Geometry check sheet. Reference: the model listing, model coordinates, mm. Face numbers are marked on the shaded views. A direction names the side the tool comes from. Round coordinates to 2 decimals unless told otherwise and drop trailing zeros. Loops run counter-clockwise (first coordinate to the right, second up) from the corner with the lowest first, then second, coordinate; pieces in that order, holes last.
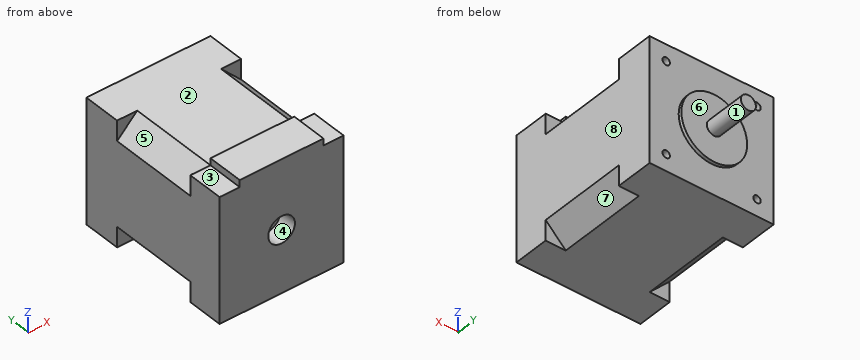
```python
from build123d import *

# Parameters (mm, degrees)
SKETCH1_W               = 41.45
SKETCH1_H               = 41.45
BOSS_EXTRUDE1_DEPTH     = 54.6
SKETCH2_R               = 11
BOSS_EXTRUDE2_DEPTH     = 1.1
SKETCH3_R               = 2.5
BOSS_EXTRUDE3_DEPTH     = 14
BOSS_EXTRUDE4_DEPTH     = 12
SKETCH5_R               = 1.25
CUT_EXTRUDE1_DEPTH      = 12
MIRROR2_COPY_1_SKETCH_R = 1.25
MIRROR2_COPY_1_DEPTH    = 12
CUT_EXTRUDE2_DEPTH      = 30
MIRROR4_COPY_1_DEPTH    = 30
SKETCH10_R              = 4.45
CUT_EXTRUDE3_DEPTH      = 6


with BuildPart() as part:
    # Sketch1 → Boss-Extrude1 (new body)
    with BuildSketch(Plane(origin=(0, 0, 0), x_dir=(1, 0, 0), z_dir=(0, 1, 0))):
        Rectangle(SKETCH1_W, SKETCH1_H)
    extrude(amount=BOSS_EXTRUDE1_DEPTH)

    # Sketch2 → Boss-Extrude2 (add)
    with BuildSketch(Plane(origin=(0, 54.6, 0), x_dir=(1, 0, 0), z_dir=(0, 1, 0))):
        Circle(SKETCH2_R)
    extrude(amount=BOSS_EXTRUDE2_DEPTH)

    # Sketch3 → Boss-Extrude3 (add)
    with BuildSketch(Plane(origin=(0, 55.7, 0), x_dir=(1, 0, 0), z_dir=(0, 1, 0))):
        Circle(SKETCH3_R)
    extrude(amount=BOSS_EXTRUDE3_DEPTH)

    # Sketch4 → Boss-Extrude4 (add)
    with BuildSketch(Plane.XZ):
        Polygon((0, 20.725), (14, 20.725), (14, 23.025), (-14, 23.025), (-14, 20.725), align=None)
    extrude(amount=-BOSS_EXTRUDE4_DEPTH)

    # Sketch5 → Cut-Extrude1 (cut)
    with BuildSketch(Plane(origin=(0, 54.6, 0), x_dir=(1, 0, 0), z_dir=(0, 1, 0))):
        with Locations((15.175, 15.175)):
            Circle(SKETCH5_R)
    cut_extrude1 = extrude(amount=-CUT_EXTRUDE1_DEPTH, mode=Mode.SUBTRACT)

    # Mirror1: Cut-Extrude1 across plane
    add(cut_extrude1.mirror(Plane.XY), mode=Mode.SUBTRACT)

    # Mirror2: Cut-Extrude1 across plane
    add(cut_extrude1.mirror(Plane(origin=(0, 0, 0), x_dir=(0, 0, 1), z_dir=(1, 0, 0))), mode=Mode.SUBTRACT)

    # Mirror2 copy 1 sketch → Mirror2 copy 1 (cut)
    with BuildSketch(Plane(origin=(0, 54.6, 0), x_dir=(-1, 0, 0), z_dir=(0, 1, 0))):
        with Locations((15.175, 15.175)):
            Circle(MIRROR2_COPY_1_SKETCH_R)
    extrude(amount=-MIRROR2_COPY_1_DEPTH, mode=Mode.SUBTRACT)

    # Sketch8 → Cut-Extrude2 (cut)
    with BuildSketch(Plane(origin=(0, 12, 0), x_dir=(1, 0, 0), z_dir=(0, 1, 0))):
        Polygon((-20.725, 14), (-20.725, 20.725), (-14, 20.725), align=None)
    cut_extrude2 = extrude(amount=CUT_EXTRUDE2_DEPTH, mode=Mode.SUBTRACT)

    # Mirror3: Cut-Extrude2 across plane
    add(cut_extrude2.mirror(Plane(origin=(0, 0, 0), x_dir=(0, 0, 1), z_dir=(1, 0, 0))), mode=Mode.SUBTRACT)

    # Mirror4: Cut-Extrude2 across plane
    add(cut_extrude2.mirror(Plane.XY), mode=Mode.SUBTRACT)

    # Mirror4 copy 1 sketch → Mirror4 copy 1 (cut)
    with BuildSketch(Plane(origin=(0, 12, 0), x_dir=(-1, 0, 0), z_dir=(0, 1, 0))):
        Polygon((-20.725, 14), (-20.725, 20.725), (-14, 20.725), align=None)
    extrude(amount=MIRROR4_COPY_1_DEPTH, mode=Mode.SUBTRACT)

    # Sketch10 → Cut-Extrude3 (cut)
    with BuildSketch(Plane.XZ):
        Circle(SKETCH10_R)
    extrude(amount=-CUT_EXTRUDE3_DEPTH, mode=Mode.SUBTRACT)


solid = part.part
```
1) Scan lines: line 1 along Y through (x, z) = (19, -18); line 2 along Y through (x, z) = (11, -15.5); line 3 along Z through (x, y) = (-11, 15) (3 decimals). Record each from-to range of solid material in increasing order.
Report:
line 1: y = 0 to 12, 42 to 54.6
line 2: y = 0 to 54.6
line 3: z = -20.725 to 20.725
2) Gauge pin test, flat ends, axial feed: pin 1 (7.5 mm diameter, centred on x = 16.5, z = 18, fed in from +Y); pin 2 (2 mm diameter, centred on x = 17, y = 6.5, fed in from +Z) (3 decimals); pin 3 (2.5 mm diameter, centred on x = 0.5, z = 0, fed in from -Y). Record the tip position at first contact, or that the pin passes through.
Report:
pin 1: stops at y = 54.6
pin 2: stops at z = 20.725
pin 3: stops at y = 6
3) Sectioned sample at A-A, the plane y = 5. Record the cut outline in (x, z) (3 decimals).
Report:
outline: (-20.725, -20.725) - (20.725, -20.725) - (20.725, 20.725) - (14, 20.725) - (14, 23.025) - (-14, 23.025) - (-14, 20.725) - (-20.725, 20.725) - close; hole circle Ø8.9 at (0, 0)
4) Sectioned sample at C-C, the plane z = 0. Record the cut outline in (x, y) (3 decimals).
Report:
outline: (-20.725, 0) - (-4.45, 0) - (-4.45, 6) - (4.45, 6) - (4.45, 0) - (20.725, 0) - (20.725, 54.6) - (11, 54.6) - (11, 55.7) - (2.5, 55.7) - (2.5, 69.7) - (-2.5, 69.7) - (-2.5, 55.7) - (-11, 55.7) - (-11, 54.6) - (-20.725, 54.6) - close
5) Sectioned sample at B-B, the plane x = 0. Record the cut outline in (y, z) (3 decimals), then the cut area to 3 significant figures.
Report:
outline: (0, -20.725) - (54.6, -20.725) - (54.6, -11) - (55.7, -11) - (55.7, -2.5) - (69.7, -2.5) - (69.7, 2.5) - (55.7, 2.5) - (55.7, 11) - (54.6, 11) - (54.6, 20.725) - (12, 20.725) - (12, 23.025) - (0, 23.025) - (0, 4.45) - (6, 4.45) - (6, -4.45) - (0, -4.45) - close
area: 2,330 mm2
6) Sectioned sample at D-D, the plane y = 25.5. Record the cut outline in (x, z) (3 decimals), then the cut area to 3 significant figures.
Report:
outline: (-20.725, -14) - (-14, -20.725) - (14, -20.725) - (20.725, -14) - (20.725, 14) - (14, 20.725) - (-14, 20.725) - (-20.725, 14) - close
area: 1,630 mm2
7) Mould release check, pull along Y, two halves, no side actions. Record for the marked faces 6, 7 and 8: +Y half, -Y half, draft (parallel to the pull), parting line (faces both ways), or undercut.
Report:
face 6: +Y half
face 7: undercut
face 8: draft
8) Access from +Z, -Z, +X, -X, +Y, -Y to the whole of each face (thin tool, end or side, straight path). Record for the marked faces 1, 2, 3, 4 and 5.
Report:
face 1: +Y
face 2: +Z, +X, -X, +Y
face 3: +Z, -X, +Y, -Y
face 4: -Y
face 5: +Z, -X
